Here's how the part is built. I have some questions about the finished solid (model axes, mm). A direction names the side the tool comes from. Give positions to 0.01 mm unless a question says otherwise; leave off trailing zeros. Order: outer loops, then holes, each group sorted by start corner. A loop starts at its lowest first (then second) coordinate and runs counter-clockwise, first axis right, second up.
from build123d import *

# Parameters (mm, degrees)
F1_DEPTH = 177.8
F3_DEPTH = 98.553
F5_DEPTH = 52.452


with BuildPart() as f1:
    # F0 (on Top) → F1 (new body)
    with BuildSketch(Plane.XY):
        with BuildLine():
            Line((52.451, 0), (8.001, 0))
            ThreePointArc((8.001, 0), (2.343439, -2.343439), (0, -8.001))
            Line((0, -8.001), (0, -98.552))
            Line((0, -98.552), (4.7752, -98.552))
            Line((4.7752, -98.552), (4.7752, -7.3152))
            ThreePointArc((4.7752, -7.3152), (5.519149, -5.519149), (7.3152, -4.7752))
            Line((7.3152, -4.7752), (52.451, -4.7752))
            Line((52.451, -4.7752), (52.451, 0))
        make_face()
    extrude(amount=F1_DEPTH)

    # F2 (on face) → F3 (cut, through all)
    with BuildSketch(Plane(origin=(0, 0, 0), x_dir=(-1, 0, 0), z_dir=(0, 1, 0))):
        with BuildLine():
            ThreePointArc((-52.451, 173.736), (-51.260682, 176.609682), (-48.387, 177.8))
            Line((-48.387, 177.8), (-52.451, 177.8))
            Line((-52.451, 177.8), (-52.451, 173.736))
        make_face()
        with BuildLine():
            ThreePointArc((-48.387, 0), (-51.260682, 1.190318), (-52.451, 4.064))
            Line((-52.451, 4.064), (-52.451, 0))
            Line((-52.451, 0), (-48.387, 0))
        make_face()
        with BuildLine():
            Line((-35.306, 50.6984), (-35.306, 36.730615))
            ThreePointArc((-35.306, 36.730615), (-39.864123, 32.092579), (-41.529, 25.8064))
            ThreePointArc((-41.529, 25.8064), (-22.542821, 14.771277), (-22.352, 36.730615))
            Line((-22.352, 36.730615), (-22.352, 50.6984))
            ThreePointArc((-22.352, 50.6984), (-28.829, 57.1754), (-35.306, 50.6984))
        make_face()
        with BuildLine():
            Line((-35.306, 153.797), (-35.306, 139.829215))
            ThreePointArc((-35.306, 139.829215), (-39.864123, 135.191179), (-41.529, 128.905))
            ThreePointArc((-41.529, 128.905), (-22.542821, 117.869877), (-22.352, 139.829215))
            Line((-22.352, 139.829215), (-22.352, 153.797))
            ThreePointArc((-22.352, 153.797), (-28.829, 160.274), (-35.306, 153.797))
        make_face()
    extrude(amount=-F3_DEPTH, mode=Mode.SUBTRACT)

    # F4 (on face) → F5 (cut, through all)
    with BuildSketch(Plane(origin=(0, 0, 0), x_dir=(0, -1, 0), z_dir=(-1, 0, 0))):
        with BuildLine():
            ThreePointArc((92.15891, 119.504907), (94.091728, 111.930262), (94.742, 104.14))
            Line((94.742, 104.14), (94.742, 114.935))
            ThreePointArc((94.742, 114.935), (94.051539, 117.55971), (92.15891, 119.504907))
        make_face()
        with BuildLine():
            Line((54.229, 91.059), (54.229, 104.14))
            ThreePointArc((54.229, 104.14), (52.369128, 108.630128), (47.879, 110.49))
            Line((47.879, 110.49), (26.422334, 110.49))
            ThreePointArc((26.422334, 110.49), (18.705275, 104.824536), (25.059111, 97.663583))
            Line((25.059111, 97.663583), (32.901534, 97.558367))
            Line((32.901534, 97.558367), (41.283534, 95.742102))
            Line((41.283534, 95.742102), (41.283534, 91.391388))
            ThreePointArc((41.283534, 91.391388), (47.585751, 84.584134), (54.229, 91.059))
        make_face()
        with BuildLine():
            ThreePointArc((54.483, 57.635603), (83.279054, 73.385138), (94.742, 104.14))
            ThreePointArc((94.742, 104.14), (94.091728, 111.930262), (92.15891, 119.504907))
            ThreePointArc((92.15891, 119.504907), (90.835528, 120.074428), (89.408, 120.269))
            Line((89.408, 120.269), (71.628, 120.269))
            ThreePointArc((71.628, 120.269), (67.856292, 118.706708), (66.294, 114.935))
            Line((66.294, 114.935), (66.294, 104.14))
            Line((66.294, 104.14), (72.771, 104.14))
            Line((72.771, 104.14), (79.248, 104.14))
            Line((79.248, 104.14), (79.248, 107.95))
            Line((79.248, 107.95), (83.107304, 107.95))
            ThreePointArc((83.107304, 107.95), (74.209487, 80.380476), (47.752, 68.58))
            Line((47.752, 68.58), (47.373243, 68.58))
            ThreePointArc((47.373243, 68.58), (42.883115, 66.720128), (41.023243, 62.23))
            Line((41.023243, 62.23), (41.023243, 48.564316))
            ThreePointArc((41.023243, 48.564316), (47.665111, 41.660113), (54.483, 48.390552))
            Line((54.483, 48.390552), (54.483, 57.635603))
        make_face()
        with BuildLine():
            Line((72.771, 104.14), (66.294, 104.14))
            ThreePointArc((66.294, 104.14), (72.771, 97.663), (79.248, 104.14))
            Line((79.248, 104.14), (72.771, 104.14))
        make_face()
        with BuildLine():
            Line((98.552, 0), (98.552, 48.26))
            ThreePointArc((98.552, 48.26), (84.416973, 14.135027), (50.292, 0))
            Line((50.292, 0), (98.552, 0))
        make_face()
        with BuildLine():
            Line((98.552, 177.8), (50.292, 177.8))
            ThreePointArc((50.292, 177.8), (84.416973, 163.664973), (98.552, 129.54))
            Line((98.552, 129.54), (98.552, 177.8))
        make_face()
    extrude(amount=-F5_DEPTH, mode=Mode.SUBTRACT)


solid = f1.part
Q1. If we section it at B-B on x = 20: List the corners of the cut face in (y, z) for me.
Filled sheet:
outline: (-4.78, 0) - (0, 0) - (0, 16.68) - (-4.78, 16.68) - close; (-4.78, 34.94) - (0, 34.94) - (0, 119.78) - (-4.78, 119.78) - close; (-4.78, 138.03) - (0, 138.03) - (0, 177.8) - (-4.78, 177.8) - close
Q2. I'm going to push flat-ended pins straight in: P1, Ø10, axis at x = 7.5, y = -56, coming from the -Z side; P2, Ø1.9, axis at x = 1.5, z = 107, coming from the +Y side; P3, Ø10, axis at x = 46, z = 146, coming from the -Y side. Where does each tip first touch, or does it pass through?
Filled sheet:
P1: stops at z = 0.02
P2: stops at y = -2.24
P3: stops at y = -4.78
Q3. If we section it at A-A on y = -35.5: List the corners of the cut face in (x, z) for me.
Filled sheet:
outline: (0, 0) - (4.78, 0) - (4.78, 97) - (0, 97) - close; (0, 110.49) - (4.78, 110.49) - (4.78, 177.8) - (0, 177.8) - close
Q4. For faces 4 (the face through (30, -4.775, 88)), 5 (the face through (2, -54.483, 53)), 6 (the face through (35.306, -2, 147)), 7 (the face through (51.29, -2.35, 176.58)), which set-ups out of +Z, -Z, +X, -X, +Y, -Y let a thin tool reach every point of the face, with its end or its side?
Filled sheet:
face 4: +Z, -Z, +X, -Y
face 5: +X, -X
face 6: +Y, -Y
face 7: +Z, +X, +Y, -Y
Q5. I need wall thicknesses on L1, parallel to Y at x = 2, z = 104; L2, parallel to X at y = -40, z = 165.5; L3, parallel to Y at x = 19.5, z = 155. Which ranges of each line are inside material? Lowest first, please.
Filled sheet:
L1: y = -98.55 to -94.74, -83.31 to -79.25, -66.3 to -54.23, -18.67 to -2.71
L2: x = 0 to 4.78
L3: y = -4.78 to 0
Q6. Thinking about a two-plate mould opening in Z: for faces 1 (the face through (2, -98.552, 88)), 2 (the face through (2, -54.229, 98)), 3 (the face through (4, -14, 0)), which applies, released by +Z, released by -Z, zero draft, split by the parting line, or undercut?
Filled sheet:
face 1: zero draft
face 2: undercut
face 3: released by -Z
Q7. If we section it at C-C on y = -68: List the corners of the cut face in (x, z) for me, plus the area to 3 significant figures.
Filled sheet:
outline: (0, 3.37) - (4.78, 3.37) - (4.78, 61.74) - (0, 61.74) - close; (0, 74.91) - (4.78, 74.91) - (4.78, 99.76) - (0, 99.76) - close; (0, 118.85) - (4.78, 118.85) - (4.78, 174.43) - (0, 174.43) - close
area: 663 mm2
Q8. If we section it at D-D on z = 124: List the corners of the cut face in (x, y) for me, plus the area to 3 significant figures.
Filled sheet:
outline: (0, -98.55) - (4.78, -98.55) - (4.78, -7.32) arc R2.54 cw to (7.32, -4.78) - (17.11, -4.78) - (17.11, 0) - (8, 0) arc R8 ccw to (0, -8) - close; (40.54, -4.78) - (52.45, -4.78) - (52.45, 0) - (40.54, 0) - close
area: 574 mm2
